Can you work these out from the drawing? Everything is in mm from the part's minimum corner. Coordinates: 2 decimals unless noted, no trailing zeros. Loops run counter-clockwise (first coordinate to the right, second up) from the corner with the lowest first, then second, coordinate; pieces in that order, holes last.
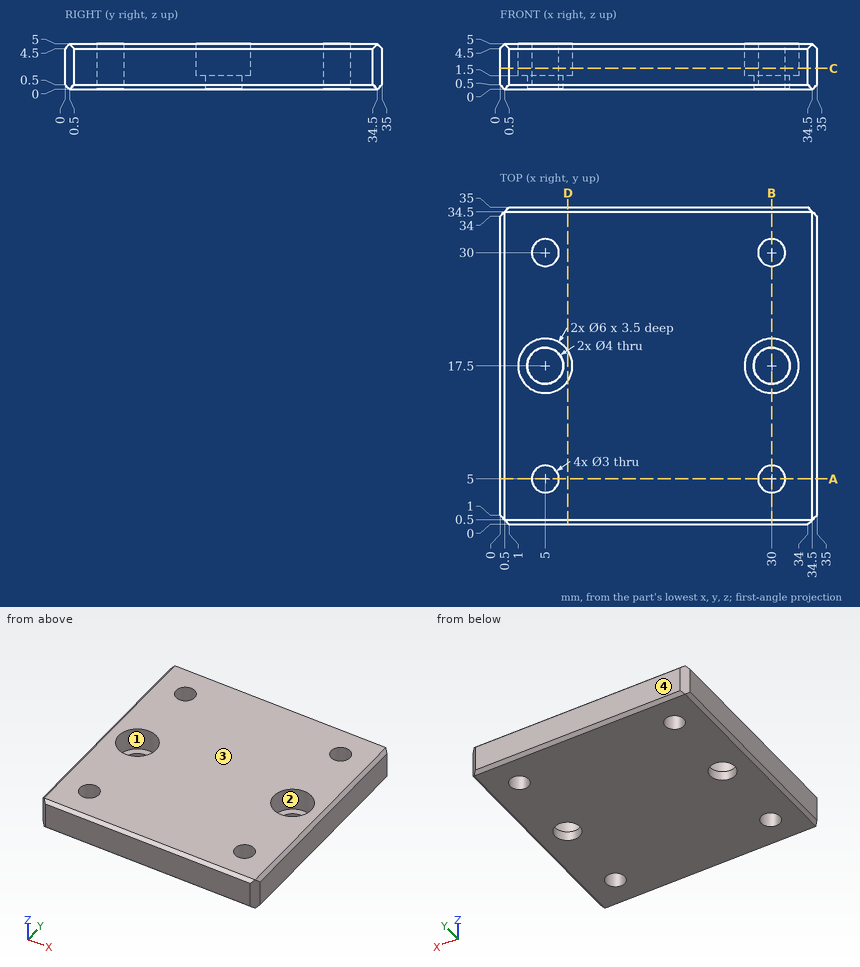
Item 1: Suppose I cut it at C-C, the plane z = 2.3. Please give me the cut outline in (x, y), plus the area to 3 significant figures.
Results are:
outline: (0, 1) - (1, 0) - (34, 0) - (35, 1) - (35, 34) - (34, 35) - (1, 35) - (0, 34) - close; hole circle Ø6 at (5, 17.5); hole circle Ø3 at (5, 5); hole circle Ø3 at (5, 30); hole circle Ø6 at (30, 17.5); hole circle Ø3 at (30, 5); hole circle Ø3 at (30, 30)
area: 1,140 mm2
Item 2: We'd pull the mould along Y, two halves only. Please class the marked faces 1, 2, 3 and 4: +Y half, -Y half, draft (parallel to the pull), parting line (faces both ways), or undercut.
Results are:
face 1: undercut
face 2: undercut
face 3: draft
face 4: +Y half
Item 3: Suppose I cut it at B-B, the plane x = 30. Please give me the cut outline in (y, z).
Results are:
outline: (0, 0.5) - (0.5, 0) - (3.5, 0) - (3.5, 5) - (0.5, 5) - (0, 4.5) - close; (6.5, 0) - (15.5, 0) - (15.5, 1.5) - (14.5, 1.5) - (14.5, 5) - (6.5, 5) - close; (19.5, 0) - (28.5, 0) - (28.5, 5) - (20.5, 5) - (20.5, 1.5) - (19.5, 1.5) - close; (31.5, 0) - (34.5, 0) - (35, 0.5) - (35, 4.5) - (34.5, 5) - (31.5, 5) - close
Item 4: I need wall thicknesses on line 1 along Y through (x, z) = (30, 3.4); line 2 along Y through (x, z) = (30, 0.65); line 3 along X through (y, z) = (17.5, 0.6). Which ranges of each line are inside material? Lowest first, please.
Results are:
line 1: y = 0 to 3.5, 6.5 to 14.5, 20.5 to 28.5, 31.5 to 35
line 2: y = 0 to 3.5, 6.5 to 15.5, 19.5 to 28.5, 31.5 to 35
line 3: x = 0 to 3, 7 to 28, 32 to 35
Item 5: Suppose I cut it at A-A, the plane y = 5. Please give me the cut outline in (x, z).
Results are:
outline: (0, 0.5) - (0.5, 0) - (3.5, 0) - (3.5, 5) - (0.5, 5) - (0, 4.5) - close; (6.5, 0) - (28.5, 0) - (28.5, 5) - (6.5, 5) - close; (31.5, 0) - (34.5, 0) - (35, 0.5) - (35, 4.5) - (34.5, 5) - (31.5, 5) - close
Item 6: Suppose I cut it at D-D, the plane x = 7.5. Please give me the cut outline in (y, z), plus the area to 3 significant figures.
Results are:
outline: (0, 0.5) - (0.5, 0) - (34.5, 0) - (35, 0.5) - (35, 4.5) - (34.5, 5) - (19.16, 5) - (19.16, 1.5) - (15.84, 1.5) - (15.84, 5) - (0.5, 5) - (0, 4.5) - close
area: 163 mm2
Item 7: I'm going to push a flat-ended pin straight in: P1, Ø3, axis at x = 31, y = 18, coming from the +Z side. Where does the tip first touch, or does it pass through?
Results are:
P1: stops at z = 1.5
